Input: part model. Units: mm. Frame: model coordinates. A direction names the side the tool comes from. Coordinates: 2 decimals unless noted, no trailing zeros. Write each loop counter-clockwise with the first axis right and the second up, starting at its lowest first coordinate (ties: lowest second). Pieces come first, ordered by that corner, then holes. Notation, with made-up numbers: (74.25, 37) - (112.25, 37) arc R28 cw to (112.25, 55) - close; hole circle Ø11 at (-2, 86.5). An arc over 180 degrees is marked (long way). Put each result on its own line as item: value. Start each with the question number.
1. Access query for faces 4 (the flat face through (-10, 0, -5)), 5 (the cylindrical face through (-0.88, 24.08, 19.98)), 6 (the flat face through (-15, 18, 3)). Directions: +Z, -Z, +X, -X, +Y, -Y. A direction counts if a zero-diameter tool reaches every point of the face in a straight line with its end or side. Return the directions, or none.
2. Pin query (flat end, axial travel): pin 1 (1.5 mm diameter, centred on x = 11, y = -26.5, fed in from -Z); pin 2 (2 mm diameter, centred on y = -19, z = -2.5, fed in from -X); pin 3 (6 mm diameter, centred on y = -24, z = -11, fed in from -X); pin 4 (2 mm diameter, centred on x = -1, y = 19.5, fed in from +Z). Return the tip coordinate at first contact, or that it passes through.
3. Cut plane C-C, the plane z = 0. Return loops of the section in (x, y), and give its area (3 significant figures).
4. Cut plane D-D, the plane y = 25.5. Return loops of the section in (x, z), and give its area (3 significant figures).
5. Cut plane A-A, the plane x = -12. Return loops of the section in (y, z), and give its area (3 significant figures).
6. Pull-direction query (Y, two-part tool) for faces 1 (the cylindrical face through (-12.65, 9.13, -8.06)), 2 (the cylindrical face through (10.74, -1.48, 2.38)), 3 (the flat face through (0, 30, 0)); classes: released by +Y, released by -Y, zero draft, split by the parting line, or undercut.
7. Line query: line 1 (Y direction, x = -12, z = -1); line 2 (Y direction, x = -12, z = -15.5); line 3 (X direction, y = 19.5, z = 11.5). Output: solid intervals per line, ascending.
8. Cut plane B-B, the plane x = 0. Return loops of the section in (y, z), and give its area (3 significant figures).
from build123d import *


with BuildPart() as part:
    # SK_EStop → EStop (revolve)
    with BuildSketch(Plane.XY, mode=Mode.PRIVATE) as estop_sk:
        Polygon((0, -45), (15, -45), (15, -3), (11, -3), (11, 0), (15, 0), (15, 18), (20, 18), (20, 30), (0, 30), align=None)
    revolve(estop_sk.sketch.rotate(Axis((0, -50, 0), (0, 1, 0)), 90), axis=Axis((0, -50, 0), (0, 1, 0)))


solid = part.part
Report:
1. face 4: none
1. face 5: +Y, -Y
1. face 6: -Y
2. pin 1: stops at z = -10.95
2. pin 2: stops at x = -14.92
2. pin 3: stops at x = -12.69
2. pin 4: stops at z = 20
3. outline: (-20, 18) - (-15, 18) - (-15, 0) - (-11, 0) - (-11, -3) - (-15, -3) - (-15, -45) - (15, -45) - (15, -3) - (11, -3) - (11, 0) - (15, 0) - (15, 18) - (20, 18) - (20, 30) - (-20, 30) - close
3. area: 2,350 mm^2
4. outline: circle Ø40 at (0, 0)
4. area: 1,260 mm^2
5. outline: (-45, -9) - (-3, -9) - (-3, 9) - (-45, 9) - close; (0, -9) - (18, -9) - (18, -16) - (30, -16) - (30, 16) - (18, 16) - (18, 9) - (0, 9) - close
5. area: 1,460 mm^2
6. face 1: zero draft
6. face 2: undercut
6. face 3: released by +Y
7. line 1: y = -45 to -3, 0 to 30
7. line 2: y = 18 to 30
7. line 3: x = -16.36 to 16.36
8. outline: (-45, -15) - (-3, -15) - (-3, -11) - (0, -11) - (0, -15) - (18, -15) - (18, -20) - (30, -20) - (30, 20) - (18, 20) - (18, 15) - (0, 15) - (0, 11) - (-3, 11) - (-3, 15) - (-45, 15) - close
8. area: 2,350 mm^2
